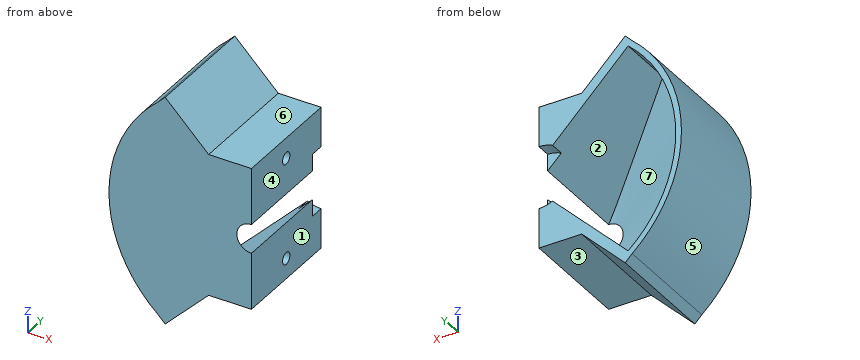
```python
from build123d import *

# Parameters (mm, degrees)
REVOLVE1_ANGLE           = 90
REVOLVE1_OTHER_WAY_ANGLE = 90
BOSS_EXTRUDE3_DEPTH      = 50.8
CUT_EXTRUDE1_REACH       = 105.175
BOSS_EXTRUDE4_DEPTH      = 50.8
SKETCH6_R                = 13.97
CUT_EXTRUDE2_DEPTH       = 6.35
SKETCH7_R                = 2.665
CUT_EXTRUDE3_DEPTH       = 8.89


with BuildPart() as part:
    # Sketch1 → Revolve1 (revolve)
    with BuildSketch(Plane.XY):
        Polygon((-63.5, 50.8), (-63.5, 0), (-6.477, 0), (-60.96, 25.405840139), (-60.96, 50.8), align=None)
    revolve(axis=Axis((0, 0, 0), (0, 1, 0)), revolution_arc=REVOLVE1_ANGLE)

    # Sketch1 → Revolve1 other way (revolve)
    with BuildSketch(Plane.XY):
        Polygon((-63.5, 50.8), (-63.5, 0), (-6.477, 0), (-60.96, 25.405840139), (-60.96, 50.8), align=None)
    revolve(axis=Axis((0, 0, 0), (0, -1, 0)), revolution_arc=REVOLVE1_OTHER_WAY_ANGLE)

    # Sketch4 → Boss-Extrude3 (add)
    with BuildSketch(Plane(origin=(0, 0, 0), x_dir=(-1, 0, 0), z_dir=(0, -1, 0))):
        Polygon((19.05, 31.75), (0, 31.75), (0, 6.477), (19.05, 25.527), align=None)
        Polygon((19.05, -25.527), (0, -6.477), (0, -31.75), (19.05, -31.75), align=None)
    extrude(amount=-BOSS_EXTRUDE3_DEPTH)

    # Sketch4<3> → Cut-Extrude1 (cut, up to next)
    with BuildSketch(Plane(origin=(0, 0, 0), x_dir=(-1, 0, 0), z_dir=(0, -1, 0)), mode=Mode.PRIVATE) as cut_extrude1_sk1:
        with BuildLine():
            Line((0, 63.5), (0, 31.75))
            Line((0, 31.75), (19.05, 31.75))
            Line((19.05, 31.75), (19.05, 25.527))
            Line((19.05, 25.527), (41.545840095, 48.022840095))
            ThreePointArc((41.545840095, 48.022840095), (22.16753994, 59.505043257), (0, 63.5))
        make_face()
    cut_extrude1_tool1 = extrude(cut_extrude1_sk1.sketch, amount=-CUT_EXTRUDE1_REACH, mode=Mode.PRIVATE) & part.part
    # Sketch4<3> → Cut-Extrude1 (cut, up to next)
    with BuildSketch(Plane(origin=(0, 0, 0), x_dir=(-1, 0, 0), z_dir=(0, -1, 0)), mode=Mode.PRIVATE) as cut_extrude1_sk2:
        with BuildLine():
            Line((19.05, -31.75), (0, -31.75))
            Line((0, -31.75), (0, -63.5))
            ThreePointArc((0, -63.5), (22.16753994, -59.505043257), (41.545840095, -48.022840095))
            Line((41.545840095, -48.022840095), (19.05, -25.527))
            Line((19.05, -25.527), (19.05, -31.75))
        make_face()
    cut_extrude1_tool2 = extrude(cut_extrude1_sk2.sketch, amount=-CUT_EXTRUDE1_REACH, mode=Mode.PRIVATE) & part.part
    add(cut_extrude1_tool1.solids().sort_by_distance((-16.601878, 0, -46.365556))[0], mode=Mode.SUBTRACT)
    add(cut_extrude1_tool2.solids().sort_by_distance((-16.601878, 0, 46.365556))[0], mode=Mode.SUBTRACT)

    # Sketch5 → Boss-Extrude4 (add)
    with BuildSketch(Plane.XZ):
        Polygon((-41.545840095, 48.022840095), (-38.434340095, 51.134340095), (-19.05, 31.75), (-19.05, 25.527), align=None)
        Polygon((-41.545840095, -48.022840095), (-38.434340095, -51.134340095), (-19.05, -31.75), (-19.05, -25.527), align=None)
    extrude(amount=-BOSS_EXTRUDE4_DEPTH)

    # Sketch6 → Cut-Extrude2 (cut)
    with BuildSketch(Plane(origin=(0, 50.8, 0), x_dir=(1, 0, 0), z_dir=(0, 1, 0))):
        Circle(SKETCH6_R)
    extrude(amount=-CUT_EXTRUDE2_DEPTH, mode=Mode.SUBTRACT)

    # Sketch7 → Cut-Extrude3 (cut)
    with BuildSketch(Plane(origin=(0, 0, 0), x_dir=(0, 0, -1), z_dir=(1, 0, 0))):
        with Locations((-22.575, 25.4)):
            Circle(SKETCH7_R)
        with Locations((22.575, 25.4)):
            Circle(SKETCH7_R)
    extrude(amount=-CUT_EXTRUDE3_DEPTH, mode=Mode.SUBTRACT)


solid = part.part
```
For this review, take the finished solid that the model builds, in its own axes (mm). Face numbers are marked on the shaded views. A direction names the side the tool comes from. Give positions to 0.01 mm unless a question says otherwise; leave off trailing zeros. Order: outer loops, then holes, each group sorted by start corner. A loop starts at its lowest first (then second) coordinate and runs counter-clockwise, first axis right, second up.
1) Take a section at D-D (y = 7). Give the boundary of the cut face in (x, z), then the cut area to 3 significant figures.
2) Insertion check: pin 1 (3 mm diameter, centred on x = -4, z = -10.5, fed in from +Y); pin 2 (8 mm diameter, centred on x = -43.5, z = -24.5, fed in from +Y); pin 3 (5 mm diameter, centred on x = -45, y = 30, fed in from -Z). Each pin has a flat end and moves straight along its axis. Give the tip position at first contact, or say it passes through.
3) The part is to be moulded in two halves that separate along Z. For the marked faces 4, 5, 6 and 7, say which applies: released by +Z, released by -Z, zero draft, split by the parting line, or undercut.
4) Wall thickness on line 1 (Z direction, x = -4, y = 25); line 2 (Z direction, x = -6, y = 25); line 3 (Z direction, x = -26.5, y = 47.5): over which ranges is each line inside the solid? List them lowest first.
5) Take a section at A-A (y = 46). Give the boundary of the cut face in (x, z), then the cut area to 3 significant figures.
6) Take a section at C-C (y = 35). Give the boundary of the cut face in (x, z), then the cut area to 3 significant figures.
7) For the marked faces 1, 2 and 3, list the 3-axis set-ups (+Z, -Z, +X, -X, +Y, -Y) from which the entire face can be reached by the end or side of a thin tool; tool diameter is ignored.
8) Take a section at B-B (z = 0). Give the boundary of the cut face in (x, y), then the cut area to 3 significant figures.
Derived:
1. outline: (-41.55, -48.02) - (-38.43, -51.13) - (-19.05, -31.75) - (0, -31.75) - (0, -6.48) - (-11.61, -18.08) arc R21.49 cw to (-11.61, 18.08) - (0, 6.48) - (0, 31.75) - (-19.05, 31.75) - (-38.43, 51.13) - (-41.55, 48.02) arc R63.5 ccw to start
1. area: 4,050 mm2
2. pin 1: stops at y = 44.45
2. pin 2: stops at y = 22.13
2. pin 3: stops at z = -47.18
3. face 4: zero draft
3. face 5: split by the parting line
3. face 6: released by +Z
3. face 7: undercut
4. line 1: z = -31.75 to -25.21, -19.94 to -10.48, 10.48 to 19.94, 25.21 to 31.75
4. line 2: z = -31.75 to -25.21, -19.94 to -12.48, 12.48 to 19.94, 25.21 to 31.75
4. line 3: z = -39.2 to -32.98, 32.98 to 39.2
5. outline: (-41.55, -48.02) - (-38.43, -51.13) - (-19.05, -31.75) - (0, -31.75) - (0, -13.97) arc R13.97 cw to (-6.09, -12.57) - (-39.74, -46.22) arc R60.96 cw to (-39.74, 46.22) - (-6.09, 12.57) arc R13.97 cw to (0, 13.97) - (0, 31.75) - (-19.05, 31.75) - (-38.43, 51.13) - (-41.55, 48.02) arc R63.5 ccw to start
5. area: 1,080 mm2
6. outline: (-41.55, -48.02) - (-38.43, -51.13) - (-19.05, -31.75) - (0, -31.75) - (0, -6.48) - (-39.74, -46.22) arc R60.96 cw to (-39.74, 46.22) - (0, 6.48) - (0, 31.75) - (-19.05, 31.75) - (-38.43, 51.13) - (-41.55, 48.02) arc R63.5 ccw to start
6. area: 1,130 mm2
7. face 1: +Z, -Z, +X, +Y, -Y
7. face 2: +Y
7. face 3: -Z, +X, +Y, -Y
8. outline: (-63.5, 0) - (-6.48, 0) - (-60.96, 25.41) - (-60.96, 50.8) - (-63.5, 50.8) - close
8. area: 821 mm2
